Verification items for the finished model (mm, model axes). Face numbers are marked on the shaded views. A direction names the side the tool comes from. Give positions to 0.01 mm unless a question says otherwise; leave off trailing zeros. Write each loop counter-clockwise with the first axis right and the second up, starting at its lowest first coordinate (ties: lowest second). Pieces come first, ordered by that corner, then holes. Notation, with made-up numbers: (-33.5, 25) - (-19.5, 25) arc R19 ccw to (-19.5, 45) - close; hole circle Ø8 at (10.25, 37). An arc over 180 degrees is marked (long way). Put each result on its own line as item: value.
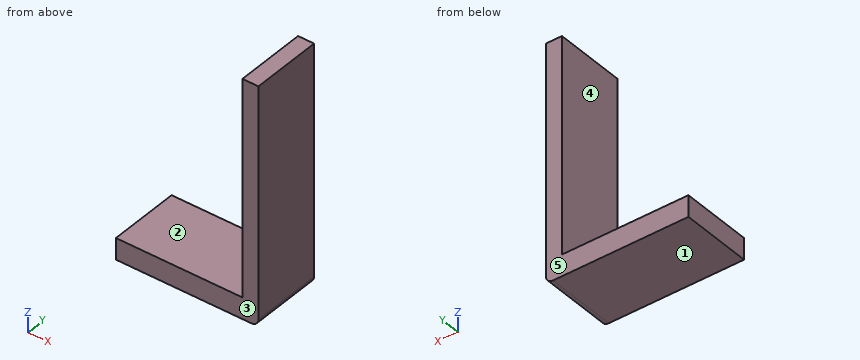
from build123d import *

# Parameters (mm, degrees)
EXTRUDE_THIN1_DEPTH = 20
SKETCH2_W           = 40
SKETCH2_H           = 20
BOSS_EXTRUDE1_DEPTH = 1.5
FILLET1_R           = 2


with BuildPart() as part:
    # Sketch1 → Extrude-Thin1 (new body)
    with BuildSketch(Plane(origin=(0, 0, 0), x_dir=(1, 0, 0), z_dir=(0, 1, 0))):
        Polygon((0, -65), (0, 0), (-40, 0), (-40, -4.5), (-4.5, -4.5), (-4.5, -65), align=None)
    extrude(amount=EXTRUDE_THIN1_DEPTH)

    # Sketch2 → Boss-Extrude1 (add)
    with BuildSketch(Plane(origin=(0, 0, 0), x_dir=(-1, 0, 0), z_dir=(0, 0, -1))):
        with Locations((20, 10)):
            Rectangle(SKETCH2_W, SKETCH2_H)
    extrude(amount=BOSS_EXTRUDE1_DEPTH)

    # Fillet1
    fillet1_edges = [part.edges().sort_by_distance(p)[0] for p in [
        (0, 10, -1.5),
    ]]
    fillet(fillet1_edges, radius=FILLET1_R)


solid = part.part
Q1. Scan lines: line 1 along X through (y, z) = (16, 10.5); line 2 along Z through (x, y) = (-28, 17.5). Record each from-to range of solid material in increasing order.
Answers follow:
line 1: x = -4.5 to 0
line 2: z = -1.5 to 4.5
Q2. Section check B-B, the plane z = 28.5. Record the cut outline in (x, y), plus the area to 3 significant figures.
Answers follow:
outline: (-4.5, 0) - (0, 0) - (0, 20) - (-4.5, 20) - close
area: 90.0 mm2
Q3. Set-up check for the marked faces 1 and 2: record each of +Z, -Z, +X, -X, +Y, -Y from which the full face is reachable in a straight line by a thin tool's end or side.
Answers follow:
face 1: -Z, +X, -X, +Y, -Y
face 2: +Z, -X, +Y, -Y
Q4. Go/stop test with flat-tipped pins: pin 1 Ø6 at (y, z) = (5.5, 41) entering from -X; pin 2 Ø3 at (x, y) = (-21, 7) entering from +Z. Record where each tip stops, or that it passes through.
Answers follow:
pin 1: stops at x = -4.5
pin 2: stops at z = 4.5
Q5. Section check A-A, the plane y = 16.5. Record the cut outline in (x, z), plus the area to 3 significant figures.
Answers follow:
outline: (-40, -1.5) - (-2, -1.5) arc R2 ccw to (0, 0.5) - (0, 65) - (-4.5, 65) - (-4.5, 4.5) - (-40, 4.5) - close
area: 511 mm2
Q6. Section check C-C, the plane x = -20.5. Record the cut outline in (y, z), plus the area to 3 significant figures.
Answers follow:
outline: (0, -1.5) - (20, -1.5) - (20, 4.5) - (0, 4.5) - close
area: 120 mm2
Q7. Release check for a two-part mould opening along Y. For the marked faces 3, 4 and 5 record: released by +Y, released by -Y, zero draft, split by the parting line, or undercut.
Answers follow:
face 3: released by -Y
face 4: zero draft
face 5: released by +Y
